The figure shows three views and two pictorial views of one solid part (mm, origin at its lowest corner). Answer the questions. A direction names the side the tool comes from. Give positions to 0.01 mm unless a question says otherwise; leave off trailing zeros. Write each loop counter-clockwise with the first axis right and the second up, starting at its lowest first coordinate (ties: lowest second). Pieces come first, ordered by that corner, then holes. Notation, with made-up numbers: M 27,36.5 L 39,36.5 A20 cw 39,49.5 Z; hole C 38.25,-38 d2. An arc over 180 degrees is marked long. Return JSON: item names as keys, results as strings.
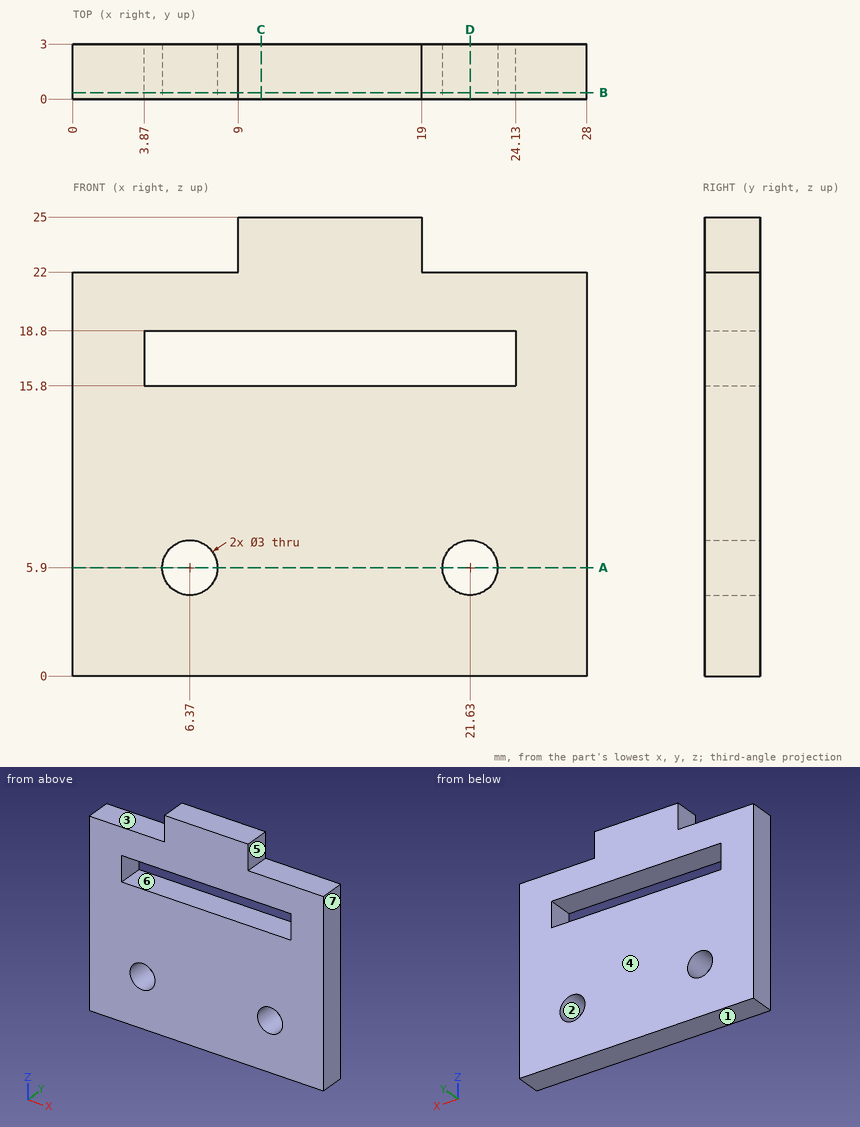
Item 1: A cutting plane is placed at A-A, the plane z = 5.9. Write down the section's boundary in (x, y).
Geometry results:
{"outline": "M 0,0 L 4.87,0 L 4.87,3 L 0,3 Z; M 7.87,0 L 20.13,0 L 20.13,3 L 7.87,3 Z; M 23.13,0 L 28,0 L 28,3 L 23.13,3 Z"}
Item 2: Given pin 1 Ø8 at (x, z) = (19.5, 4.5) entering from -Y; pin 2 Ø1.5 at (x, z) = (8.5, 17) entering from +Y; pin 3 Ø1.5 at (x, y) = (25.5, 1) entering from +Z, each flat-ended and moving along its own axis, determine where each tip first touches the part or whether it passes through.
Geometry results:
{"pin 1": "stops at y = 0", "pin 2": "passes through", "pin 3": "stops at z = 22"}
Item 3: Determine the mould class of the marked faces 1, 2, 3 and 4 for opening direction Z: +Z half, -Z half, draft (parallel to the pull), parting line (faces both ways), or undercut.
Geometry results:
{"face 1": "-Z half", "face 2": "undercut", "face 3": "+Z half", "face 4": "draft"}
Item 4: A cutting plane is placed at D-D, the plane x = 21.63. Write down the section's boundary in (y, z).
Geometry results:
{"outline": "M 0,0 L 3,0 L 3,4.4 L 0,4.4 Z; M 0,7.4 L 3,7.4 L 3,15.8 L 0,15.8 Z; M 0,18.8 L 3,18.8 L 3,22 L 0,22 Z"}
Item 5: A cutting plane is placed at B-B, the plane y = 0.35. Write down the section's boundary in (x, z), plus the area to 3 significant figures.
Geometry results:
{"outline": "M 0,0 L 28,0 L 28,22 L 19,22 L 19,25 L 9,25 L 9,22 L 0,22 Z; hole M 3.87,15.8 L 24.13,15.8 L 24.13,18.8 L 3.87,18.8 Z; hole C 6.37,5.9 d3; hole C 21.63,5.9 d3", "area": "571 mm2"}
Item 6: Find the intervals of material crossed by line 1 (X direction, y = 0.95, z = 5.9); line 2 (Z direction, x = 6.37, y = 1.95); line 3 (Z direction, x = 12, y = 2.75), in increasing order.
Geometry results:
{"line 1": "x = 0 to 4.87, 7.87 to 20.13, 23.13 to 28", "line 2": "z = 0 to 4.4, 7.4 to 15.8, 18.8 to 22", "line 3": "z = 0 to 15.8, 18.8 to 25"}
Item 7: A cutting plane is placed at C-C, the plane x = 10.25. Write down the section's boundary in (y, z), plus the area to 3 significant figures.
Geometry results:
{"outline": "M 0,0 L 3,0 L 3,15.8 L 0,15.8 Z; M 0,18.8 L 3,18.8 L 3,25 L 0,25 Z", "area": "66.0 mm2"}
Item 8: Which of the six approach directions +Z, -Z, +X, -X, +Y, -Y give full straight-line access (tool end or side, diameter ignored) to the marked faces 5, 6 and 7?
Geometry results:
{"face 5": "+Z, +X, +Y, -Y", "face 6": "+Y, -Y", "face 7": "+Z, -Z, +X, +Y, -Y"}
